```python
from build123d import *

# Parameters (mm, degrees)
SKETCH_1_R               = 2.05
EXTRUDE_1_DEPTH          = 5
EXTRUDE_2_DEPTH          = 15
CUT_EXTRUDE_1_DEPTH      = 86.775919648
CUT_EXTRUDE_1_DEPTH_BACK = 86.775919648
SKETCH_3_R               = 1.55


with BuildPart() as part:
    # 草图1 → 凸台-拉伸1 (new body)
    with BuildSketch(Plane(origin=(0, 0, 0), x_dir=(1, 0, 0), z_dir=(0, 1, 0))):
        with BuildLine():
            Line((-5.656854249, 45.343145751), (-45.343145751, 5.656854249))
            ThreePointArc((-45.343145751, 5.656854249), (-47.686291501, 0), (-45.343145751, -5.656854249))
            Line((-45.343145751, -5.656854249), (-5.656854249, -45.343145751))
            ThreePointArc((-5.656854249, -45.343145751), (0, -47.686291501), (5.656854249, -45.343145751))
            Line((5.656854249, -45.343145751), (45.343145751, -5.656854249))
            ThreePointArc((45.343145751, -5.656854249), (47.686291501, 0), (45.343145751, 5.656854249))
            Line((45.343145751, 5.656854249), (5.656854249, 45.343145751))
            ThreePointArc((5.656854249, 45.343145751), (0, 47.686291501), (-5.656854249, 45.343145751))
        make_face()
        with Locations(Location((0, 40, 0), (0, 0, 270))):
            Circle(SKETCH_1_R, mode=Mode.SUBTRACT)
        with Locations(Location((40, 0, 0), (0, 0, 270))):
            Circle(SKETCH_1_R, mode=Mode.SUBTRACT)
        with Locations(Location((0, -40, 0), (0, 0, 270))):
            Circle(SKETCH_1_R, mode=Mode.SUBTRACT)
        with Locations(Location((-40, 0, 0), (0, 0, 270))):
            Circle(SKETCH_1_R, mode=Mode.SUBTRACT)
    extrude(amount=EXTRUDE_1_DEPTH)

    # 草图2 → 凸台-拉伸2 (add)
    with BuildSketch(Plane(origin=(0, 5, 0), x_dir=(1, 0, 0), z_dir=(0, 1, 0))):
        Polygon((-24.75, 14.75), (-21.75, 14.75), (-21.75, 17.75), (21.75, 17.75), (21.75, 14.75), (24.75, 14.75), (24.75, 20.75), (-24.75, 20.75), align=None)
        Polygon((24.75, -20.75), (-24.75, -20.75), (-24.75, -14.75), (-21.75, -14.75), (-21.75, -17.75), (21.75, -17.75), (21.75, -14.75), (24.75, -14.75), align=None)
    extrude(amount=EXTRUDE_2_DEPTH)

    # 草图3 → 切除-拉伸1 (cut, two sides: drawn at the far end of the back side and taken through both)
    with BuildSketch(Plane.XY.offset(20.75).offset(-CUT_EXTRUDE_1_DEPTH_BACK)):
        with Locations((0, 13)):
            Circle(SKETCH_3_R)
    extrude(amount=CUT_EXTRUDE_1_DEPTH + CUT_EXTRUDE_1_DEPTH_BACK, mode=Mode.SUBTRACT)


solid = part.part
```
CAD build for the part. Positions are in the model's coordinates, mm. A direction names the side the tool comes from. Coordinates: 2 decimals unless noted, no trailing zeros. Order: outer loops, then holes, each group sorted by start corner. A loop starts at its lowest first (then second) coordinate and runs counter-clockwise, first axis right, second up. Notation, with made-up numbers: M 60,57.5 L 104,57.5 A28 cw 104,87.5 Z; hole C 20.5,44.25 d8. An arc over 180 degrees is marked long. Write each question's results on one line, items separated by ' | '. Start each with the question number.
Q1. Pull direction Y, two halves, no side cores. Call faces 6 (the flat face through (-1, 0, -1)), 7 (the cylindrical face through (0.83, 14.31, -19.27)), 8 (the cylindrical face through (0.83, 14.31, 19.23)), 9 (the flat face through (-21.75, 12, -16)): +Y half, -Y half, draft (parallel to the pull), parting line (faces both ways), or undercut.
Q2. Cut at D-D (y = 18.75). List the corners of the cut face in (x, z).
Q3. Flat gauge pins, fed straight in: P1, Ø3, axis at x = 0, y = 13, coming from the -Z side; P2, Ø1.8, axis at y = 9.5, z = 17.5, coming from the +X side; P3, Ø12, axis at x = -9.5, y = 2, coming from the +Z side; P4, Ø8, axis at x = 34, z = -3, coming from the +Y side. Where does each tip first touch, or does it go through?
Q4. Cut at C-C (z = -40). List the corners of the cut face in (x, y).
Q5. Which spindle directions (+Z, -Z, +X, -X, +Y, -Y) get a long thin tool onto all of the face, cutting with end or side? Do faces 1 (the flat face through (23, 12, -14.75)), 2 (the flat face through (-24.75, 12, -18)), 3 (the cylindrical face through (-47.686, 2.465, -0.088)), 4 (the cylindrical face through (47.686, 2.465, 0.088)), 5 (the flat face through (0, 11, -17.75)). Say none if no direction does.
Q6. Cut at A-A (x = 40). List the corners of the cut face in (y, z).
Q7. Cut at B-B (y = 13). List the corners of the cut face in (x, z).
Q8. Drill centre lines: probe 1 along Y at (x, z) = (0, -20.1); probe 2 along Z at (x, y) = (-18.5, 13); probe 3 along Z at (x, y) = (22, 19). Where is each one in solid material? Low to high. Write a range as from..to.
Found:
1) face 6: -Y half | face 7: undercut | face 8: undercut | face 9: draft
2) outline: M -24.75,-20.75 L 24.75,-20.75 L 24.75,-14.75 L 21.75,-14.75 L 21.75,-17.75 L -21.75,-17.75 L -21.75,-14.75 L -24.75,-14.75 Z; M -24.75,14.75 L -21.75,14.75 L -21.75,17.75 L 21.75,17.75 L 21.75,14.75 L 24.75,14.75 L 24.75,20.75 L -24.75,20.75 Z
3) P1: through | P2: x = 24.75 | P3: z = 46.88 | P4: y = 5
4) outline: M -11,0 L -2.05,0 L -2.05,5 L -11,5 Z; M 2.05,0 L 11,0 L 11,5 L 2.05,5 Z
5) face 1: +X, -X, +Y | face 2: +Z, -Z, -X, +Y | face 3: -X, +Y, -Y | face 4: +X, +Y, -Y | face 5: +Y
6) outline: M 0,-11 L 5,-11 L 5,-2.05 L 0,-2.05 Z; M 0,2.05 L 5,2.05 L 5,11 L 0,11 Z
7) outline: M -24.75,-20.75 L -1.55,-20.75 L -1.55,-17.75 L -21.75,-17.75 L -21.75,-14.75 L -24.75,-14.75 Z; M -24.75,14.75 L -21.75,14.75 L -21.75,17.75 L -1.55,17.75 L -1.55,20.75 L -24.75,20.75 Z; M 1.55,-20.75 L 24.75,-20.75 L 24.75,-14.75 L 21.75,-14.75 L 21.75,-17.75 L 1.55,-17.75 Z; M 1.55,17.75 L 21.75,17.75 L 21.75,14.75 L 24.75,14.75 L 24.75,20.75 L 1.55,20.75 Z
8) probe 1: 0..11.45, 14.55..20 | probe 2: -20.75..-17.75, 17.75..20.75 | probe 3: -20.75..-14.75, 14.75..20.75
